from build123d import *

# Parameters (mm, degrees)
F1_DEPTH = 21.59
F2_R     = 8.89
F3_R     = 8.89
F4_R     = 1.27
F5_R     = 1.27
F6_R     = 1.27
F7_R     = 8.093048
F8_DEPTH = 38.1


with BuildPart() as f1:
    # F0 (on Front) → F1 (new body)
    with BuildSketch(Plane.XZ):
        Polygon((-11.43, 0), (-22.86, 0), (-22.86, -3.830776), (23.048284, -3.830776), (22.86, 0), (11.43, 0), (0, 0), align=None)
        Polygon((-11.43, 38.1), (-11.43, 0), (0, 0), (11.43, 0), (11.43, 38.1), align=None)
    extrude(amount=F1_DEPTH)

    # F2
    f2_edges = [f1.edges().sort_by_distance(p)[0] for p in [
        (11.43, -21.59, 19.05),
    ]]
    fillet(f2_edges, radius=F2_R)

    # F3
    f3_edges = [f1.edges().sort_by_distance(p)[0] for p in [
        (-11.43, -21.59, 19.05),
        (11.43, 0, 19.05),
        (-11.43, 0, 19.05),
    ]]
    fillet(f3_edges, radius=F3_R)

    # F4
    f4_edges = [f1.edges().sort_by_distance(p)[0] for p in [
        (-22.86, -10.795, 0),
    ]]
    fillet(f4_edges, radius=F4_R)

    # F5
    f5_edges = [f1.edges().sort_by_distance(p)[0] for p in [
        (-22.86, -10.795, -3.830776),
    ]]
    fillet(f5_edges, radius=F5_R)

    # F6
    f6_edges = [f1.edges().sort_by_distance(p)[0] for p in [
        (-16.51, 0, 0),
        (0.729142, 0, -3.830776),
        (6.985, 0, 0),
        (22.86, -10.795, 0),
        (23.048284, -10.795, -3.830776),
        (17.145, -21.59, 0),
        (0.729142, -21.59, -3.830776),
        (-16.51, -21.59, 0),
    ]]
    fillet(f6_edges, radius=F6_R)

    # F7 (on face) → F8 (cut)
    with BuildSketch(Plane(origin=(0, 0, -3.830776), x_dir=(1, 0, 0), z_dir=(0, 0, -1))):
        with Locations((0, 11.323408)):
            Circle(F7_R)
    extrude(amount=-F8_DEPTH, mode=Mode.SUBTRACT)


solid = f1.part
Design review of the part built by this model. Coordinates are the model's own, in mm. A direction names the side the tool comes from. Coordinates: 2 decimals unless noted, no trailing zeros. Order: outer loops, then holes, each group sorted by start corner. A loop starts at its lowest first (then second) coordinate and runs counter-clockwise, first axis right, second up. Notation, with made-up numbers: M -2,81.5 L 35,81.5 A21 cw 35,90.5 Z; hole C 52.5,-3.5 d5. An arc over 180 degrees is marked long. Use a Markdown table: item, result.
(1) Draft analysis for pull direction X (two halves, no side actions). For faces 1 (the flat face through (-11.43, -11, 19)), 2 (the flat face through (16, -11, 0)), 3 (the cylindrical face through (-1.75, -3.42, 14.95)), state which applies: released by +X, released by -X, zero draft, split by the parting line, or undercut.
Worked answers:
| item | result |
|---|---|
| face 1 | released by -X |
| face 2 | zero draft |
| face 3 | undercut |
(2) For P1, Ø1, axis at x = -4, z = 18, coming from the -Y side; P2, Ø5, axis at y = -2.5, z = 5, coming from the -X side; P3, Ø4, axis at y = -10.5, z = 16.5, coming from the -X side, all flat-tipped, find the tip position at first contact; note any pin that passes through.
Worked answers:
| item | result |
|---|---|
| P1 | stops at y = -21.54 |
| P2 | stops at x = -10.53 |
| P3 | stops at x = -11.43 |
(3) For faces 4 (the cylindrical face through (-14.315, -21.228, -0.382)), 5 (the cylindrical face through (-14.048, -0.382, -0.362)), 6 (the cylindrical face through (14.853, -0.382, -0.362)), list the 3-axis set-ups (+Z, -Z, +X, -X, +Y, -Y) from which the entire face can be reached by the end or side of a thin tool; tool diameter is ignored.
Worked answers:
| item | result |
|---|---|
| face 4 | +Z, -X, -Y |
| face 5 | +Z, -X, +Y |
| face 6 | +Z, +X, +Y |
(4) Add section D-D (x = -16). Give the boundary of the cut face in (y, z), then the cut area to 3 significant figures.
Worked answers:
| item | result |
|---|---|
| outline | M -21.59,-2.56 A1.27 ccw -20.32,-3.83 L -1.27,-3.83 A1.27 ccw 0,-2.56 L 0,-1.27 A1.27 ccw -1.27,0 L -20.32,0 A1.27 ccw -21.59,-1.27 Z |
| area | 81.3 mm2 |
(5) Add section A-A (x = 0). Give the boundary of the cut face in (y, z).
Worked answers:
| item | result |
|---|---|
| outline | M -21.59,-2.56 A1.27 ccw -20.32,-3.83 L -19.42,-3.83 L -19.42,34.27 L -3.23,34.27 L -3.23,-3.83 L -1.27,-3.83 A1.27 ccw 0,-2.56 L 0,38.1 L -21.59,38.1 Z |
(6) Add section C-C (y = -15.75). Give the boundary of the cut face in (x, z), then the cut area to 3 significant figures.
Worked answers:
| item | result |
|---|---|
| outline | M -22.86,-2.56 A1.27 ccw -21.59,-3.83 L -6.78,-3.83 L -6.78,34.27 L 6.78,34.27 L 6.78,-3.83 L 21.71,-3.83 A1.27 ccw 22.98,-2.5 L 22.92,-1.21 A1.27 ccw 21.65,0 L 10.89,0 L 10.89,38.1 L -10.89,38.1 L -10.89,0 L -21.59,0 A1.27 ccw -22.86,-1.27 Z |
| area | 488 mm2 |
(7) Wall thickness on probe 1 along Y at (x, z) = (0, 22); probe 2 along Z at (x, y) = (4, -12.75); probe 3 along Z at (x, y) = (19.5, -11): over which ranges is each line inside the solid? List them lowest first.
Worked answers:
| item | result |
|---|---|
| probe 1 | y = -21.59 to -19.42, -3.23 to 0 |
| probe 2 | z = 34.27 to 38.1 |
| probe 3 | z = -3.83 to 0 |
(8) Add section B-B (z = 9). Give the boundary of the cut face in (x, y), then the cut area to 3 significant figures.
Worked answers:
| item | result |
|---|---|
| outline | M -11.43,-12.7 A8.89 ccw -2.54,-21.59 L 2.54,-21.59 A8.89 ccw 11.43,-12.7 L 11.43,-8.89 A8.89 ccw 2.54,0 L -2.54,0 A8.89 ccw -11.43,-8.89 Z; hole C 0,-11.32 d16.19 |
| area | 220 mm2 |
